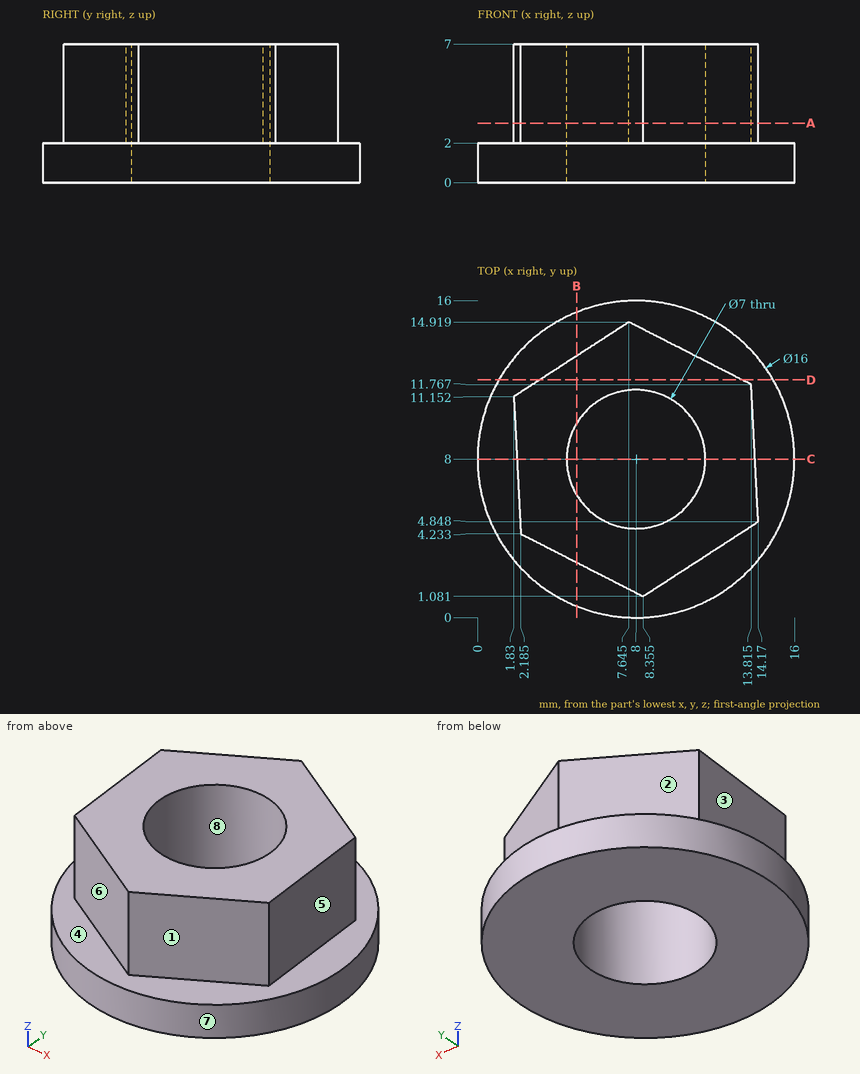
Geometry: see drawing. Coordinates: mm, zero at the bounding-box minimum. A direction names the side the tool comes from. Round coordinates to 2 decimals unless told otherwise and drop trailing zeros. Order: outer loops, then holes, each group sorted by start corner. A loop starts at its lowest first (then second) coordinate and runs counter-clockwise, first axis right, second up. Notation, with made-up numbers: (-9.75, 81) - (-2.75, 81) arc R25 cw to (-2.75, 117) - close; hole circle Ø8 at (28, 59). An arc over 180 degrees is marked (long way). Use a Markdown table: item, result. Add a question column.
1. Section query D-D (y = 12). Return the cut outline in (x, z), then the cut area to 3 significant figures.
2. Line query: probe 1 along Y at (x, z) = (9, 1) (1 decimal); probe 2 along Y at (x, z) = (8, 3); probe 3 along Z at (x, y) = (14.5, 6.25). Output: solid intervals per line, ascending.
3. Set-up query: the marked faces 1, 2, 3, 4 and 5. Return all of +Z, -Z, +X, -X, +Y, -Y with unobstructed straight access to the full face (end or side cutting, diameter ignored); none if empty.
4. Mould query, pull axis Y, two halves, no side actions, for the marked faces 6, 7 and 8. Classes: +Y half, -Y half, draft (parallel to the pull), parting line (faces both ways), or undercut.
5. First-contact query: pin 1 (6.5 mm diameter, centred on x = 8, y = 8, fed in from +Z); pin 2 (3 mm diameter, centred on y = 14, z = 3, fed in from -X); pin 3 (1.5 mm diameter, centred on x = 4.5, z = 3, fed in from +Y); pin 4 (3 mm diameter, centred on x = 13.5, z = 2.5, fed in from +Y). Flat tips, straight axial feed; report the tip coordinate or a pass-through.
6. Section query C-C (y = 8). Return the cut outline in (x, z).
7. Section query A-A (z = 3). Return the cut outline in (x, y) (1 decimal).
8. Section query B-B (x = 5). Return the cut outline in (y, z) (1 decimal).
Derived:
| question | item | result |
|---|---|---|
| 1 | outline | (1.07, 0) - (14.93, 0) - (14.93, 2) - (13.36, 2) - (13.36, 7) - (3.14, 7) - (3.14, 2) - (1.07, 2) - close |
| 1 | area | 78.8 mm2 |
| 2 | probe 1 | 0.1 to 4.6, 11.4 to 15.9 |
| 2 | probe 2 | 1.26 to 4.5, 11.5 to 14.74 |
| 2 | probe 3 | 0 to 2 |
| 3 | face 1 | +Z, +X, -Y |
| 3 | face 2 | +Z, -X, +Y |
| 3 | face 3 | +Z, -X, -Y |
| 3 | face 4 | +Z |
| 3 | face 5 | +Z, +X, +Y |
| 4 | face 6 | -Y half |
| 4 | face 7 | parting line |
| 4 | face 8 | undercut |
| 5 | pin 1 | through |
| 5 | pin 2 | x = 1.66 |
| 5 | pin 3 | y = 13.37 |
| 5 | pin 4 | y = 14.88 |
| 6 | outline | (0, 0) - (4.5, 0) - (4.5, 7) - (1.99, 7) - (1.99, 2) - (0, 2) - close; (11.5, 0) - (16, 0) - (16, 2) - (14.01, 2) - (14.01, 7) - (11.5, 7) - close |
| 7 | outline | (1.8, 11.2) - (2.2, 4.2) - (8.4, 1.1) - (14.2, 4.8) - (13.8, 11.8) - (7.6, 14.9) - close; hole circle Ø7 at (8, 8) |
| 8 | outline | (0.6, 0) - (6.2, 0) - (6.2, 7) - (2.8, 7) - (2.8, 2) - (0.6, 2) - close; (9.8, 0) - (15.4, 0) - (15.4, 2) - (13.2, 2) - (13.2, 7) - (9.8, 7) - close |
